Here's how the part is built. I have some questions about the finished solid (model axes, mm). Give positions to 0.01 mm unless a question says otherwise; leave off trailing zeros. Order: outer loops, then holes, each group sorted by start corner. A loop starts at its lowest first (then second) coordinate and runs counter-clockwise, first axis right, second up. Notation, with made-up numbers: (29.5, 44.25) - (64.5, 44.25) arc R17 cw to (64.5, 49.25) - close; hole circle Ø8 at (80, -40). An arc over 180 degrees is marked (long way). One line per question, with ' | ' between items.
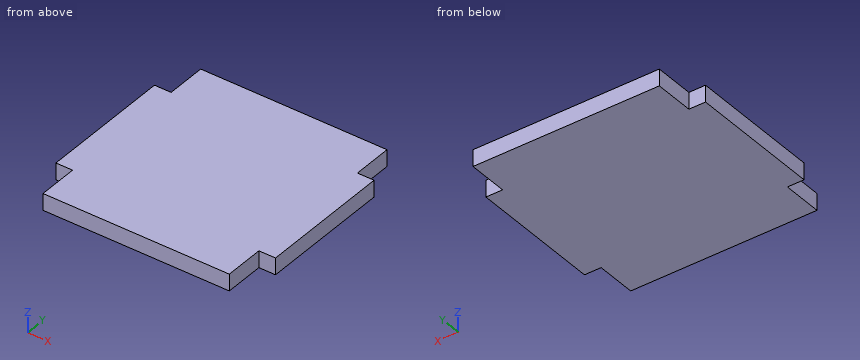
from build123d import *

# Parameters (mm, degrees)
F0_W     = 35.56
F0_H     = 40.64
F1_DEPTH = 3.175
F2_W     = 25.4
F2_H     = 3.175
F3_DEPTH = 3.175
F4_W     = 25.4
F4_H     = 3.175
F5_DEPTH = 3.175


# Not quite as in the source:
# - a length typed as a fraction of an inch, garbled in the dataset ("3 / 203.2 mm" for 3/8 in), is restored


with BuildPart() as f1:
    # F0 (on Top) → F1 (new body)
    with BuildSketch(Plane.XY):
        Rectangle(F0_W, F0_H)
    extrude(amount=F1_DEPTH)

    # F2 (on face) → F3 (join)
    with BuildSketch(Plane(origin=(-17.78, 0, 0), x_dir=(0, -1, 0), z_dir=(-1, 0, 0))):
        with Locations((0, 1.5875)):
            Rectangle(F2_W, F2_H)
    extrude(amount=F3_DEPTH)

    # F4 (on face) → F5 (join)
    with BuildSketch(Plane.YZ.offset(17.78)):
        with Locations((0, 1.5875)):
            Rectangle(F4_W, F4_H)
    extrude(amount=F5_DEPTH)


solid = f1.part
1) I want a section at B-B (y = -17.5). List the corners of the cut face in (x, z) for me (3 decimals), plus the area to 3 significant figures.
Model answer:
outline: (-17.78, 0) - (17.78, 0) - (17.78, 3.175) - (-17.78, 3.175) - close | area: 113 mm2
2) Please list where these lines run through material, in increasing order: L1, parallel to X at y = 18, z = 2.2; L2, parallel to Y at x = 19.5, z = 0.75.
Model answer:
L1: x = -17.78 to 17.78 | L2: y = -12.7 to 12.7
3) I'm going to push flat-ended pins straight in: P1, Ø1, axis at x = 20, z = 1.5, coming from the +Y side; P2, Ø1.6, axis at y = -18.5, z = 1.5, coming from the +X side; P3, Ø1, axis at y = 16.5, z = 2, coming from the -X side. Where does each tip first touch, or does it pass through?
Model answer:
P1: stops at y = 12.7 | P2: stops at x = 17.78 | P3: stops at x = -17.78
4) I want a section at A-A (z = 0.95). List the corners of the cut face in (x, y) for me (3 decimals), plus the area to 3 significant figures.
Model answer:
outline: (-20.955, -12.7) - (-17.78, -12.7) - (-17.78, -20.32) - (17.78, -20.32) - (17.78, -12.7) - (20.955, -12.7) - (20.955, 12.7) - (17.78, 12.7) - (17.78, 20.32) - (-17.78, 20.32) - (-17.78, 12.7) - (-20.955, 12.7) - close | area: 1,610 mm2
